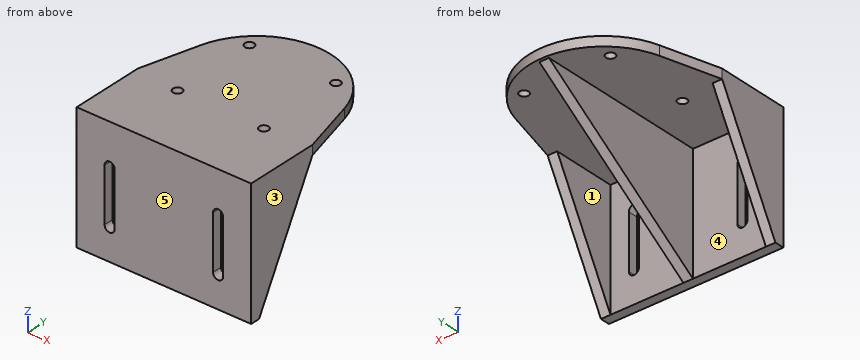
```python
from build123d import *

# Parameters (mm, degrees)
SKETCH_1_R           = 1.447765
EXTRUDE_1_DEPTH      = 3
SKETCH_2_W           = 54.999996422
SKETCH_2_H           = 3
EXTRUDE_2_DEPTH      = 37
CUT_EXTRUDE_1_DEPTH  = 3
EXTRUDE_3_DEPTH      = 3
EXTRUDE_4_DEPTH      = 1.5
EXTRUDE_4_DEPTH_BACK = 1.5


with BuildPart() as part:
    # 草图1 → 凸台-拉伸1 (new body)
    with BuildSketch(Plane.XY):
        with BuildLine():
            Line((-13.887998211, -25.578349272), (-13.887998211, -48.743989272))
            Line((-13.887998211, -48.743989272), (41.111998211, -48.743989272))
            Line((41.111998211, -48.743989272), (41.111998211, -25.578349272))
            Line((41.111998211, -25.578349272), (36.311256918, -7.661738854))
            ThreePointArc((36.311256918, -7.661738854), (13.612, 9.756013586), (-9.087256918, -7.661738854))
            Line((-9.087256918, -7.661738854), (-13.887998211, -25.578349272))
        make_face()
        Circle(SKETCH_1_R, mode=Mode.SUBTRACT)
        with Locations((27.224, 0)):
            Circle(SKETCH_1_R, mode=Mode.SUBTRACT)
        with Locations((0, -27.224)):
            Circle(SKETCH_1_R, mode=Mode.SUBTRACT)
        with Locations((27.224, -27.224)):
            Circle(SKETCH_1_R, mode=Mode.SUBTRACT)
    extrude(amount=-EXTRUDE_1_DEPTH)

    # 草图2 → 凸台-拉伸2 (add)
    with BuildSketch(Plane(origin=(0, 0, -3), x_dir=(-1, 0, 0), z_dir=(0, 0, -1))):
        with Locations((-13.612, -47.243989272)):
            Rectangle(SKETCH_2_W, SKETCH_2_H)
    extrude(amount=EXTRUDE_2_DEPTH)

    # 草图3 → 切除-拉伸1 (cut)
    with BuildSketch(Plane(origin=(0, -45.743989272, 0), x_dir=(1, 0, 0), z_dir=(0, 1, 0))):
        with BuildLine():
            Line((32.311998211, 13), (32.311998211, 30))
            ThreePointArc((32.311998211, 30), (30.711998211, 31.6), (29.111998211, 30))
            Line((29.111998211, 30), (29.111998211, 13))
            ThreePointArc((29.111998211, 13), (30.711998211, 11.4), (32.311998211, 13))
        make_face()
        with BuildLine():
            Line((-1.887998211, 30), (-1.887998211, 13))
            ThreePointArc((-1.887998211, 13), (-3.487998211, 11.4), (-5.087998211, 13))
            Line((-5.087998211, 13), (-5.087998211, 30))
            ThreePointArc((-5.087998211, 30), (-3.487998211, 31.6), (-1.887998211, 30))
        make_face()
    extrude(amount=-CUT_EXTRUDE_1_DEPTH, mode=Mode.SUBTRACT)

    # 草图4 → 凸台-拉伸3 (add)
    with BuildSketch(Plane(origin=(41.111998211, 0, 0), x_dir=(0, 0, -1), z_dir=(1, 0, 0))):
        Polygon((40, -45.743989272), (3, -25.578345661), (3, -45.743989272), align=None)
    extrude_3 = extrude(amount=-EXTRUDE_3_DEPTH)

    # 草图13 → 凸台-拉伸4 (add, two sides: drawn at the far end of the back side and taken through both)
    with BuildSketch(Plane(origin=(13.612, 0, 0), x_dir=(0, 1, 0), z_dir=(-1, 0, 0)).offset(-EXTRUDE_4_DEPTH_BACK)):
        Polygon((-45.743989272, 40), (8.756018173, 3), (-45.743989272, 3), align=None)
    extrude(amount=EXTRUDE_4_DEPTH + EXTRUDE_4_DEPTH_BACK)

    # 镜向1: 凸台-拉伸3 across plane
    add(extrude_3.mirror(Plane.ZY.offset(-13.612)))


solid = part.part
```
Can you work these out from the model? Positions are in its coordinate system, mm. Face numbers are marked on the shaded views. A direction names the side the tool comes from. Coordinates: 2 decimals unless noted, no trailing zeros. Write each loop counter-clockwise with the first axis right and the second up, starting at its lowest first coordinate (ties: lowest second). Pieces come first, ordered by that corner, then holes. Notation, with made-up numbers: (77, 1) - (114, 1) arc R37 ccw to (114, 39) - close; hole circle Ø9 at (22, 80.5). An arc over 180 degrees is marked (long way). Return JSON: item names as keys, results as strings.
Q1. I'm going to push flat-ended pins straight in: pin 1 Ø10 at (x, z) = (25, -29) entering from +Y; pin 2 Ø10 at (y, z) = (-23.5, -4.5) entering from -X; pin 3 Ø2.5 at (x, y) = (0, 0) entering from -Z; pin 4 Ø1.5 at (x, z) = (14, -33) entering from +Y. Where does each tip first touch, or does it pass through?
Computed values:
{"pin 1": "stops at y = -45.74", "pin 2": "stops at x = -13.89", "pin 3": "passes through", "pin 4": "stops at y = -34.33"}
Q2. If we section it at B-B (z = -25): Please give me the cut outline in (x, y).
Computed values:
{"outline": "(-13.89, -48.74) - (-5.09, -48.74) - (-5.09, -45.74) - (-10.89, -45.74) - (-10.89, -37.57) - (-13.89, -37.57) - close; (-1.89, -48.74) - (29.11, -48.74) - (29.11, -45.74) - (15.11, -45.74) - (15.11, -23.65) - (12.11, -23.65) - (12.11, -45.74) - (-1.89, -45.74) - close; (32.31, -48.74) - (41.11, -48.74) - (41.11, -37.57) - (38.11, -37.57) - (38.11, -45.74) - (32.31, -45.74) - close"}
Q3. On a 3-axis mill with a long thin cutter (end or side, diameter ignored), from which of +Z, -Z, +X, -X, +Y, -Y can I reach the whole of each face in a straight line? I mean the marked faces 1 and 2. Say none if no direction works.
Computed values:
{"face 1": "-Z, +Y", "face 2": "+Z, +X, -X, +Y, -Y"}
Q4. If we section it at A-A (x = 0): Please give me the cut outline in (y, z), then the cut area to 3 significant figures.
Computed values:
{"outline": "(-48.74, -40) - (-45.74, -40) - (-45.74, -3) - (-28.67, -3) - (-28.67, 0) - (-48.74, 0) - close; (-25.78, -3) - (-1.45, -3) - (-1.45, 0) - (-25.78, 0) - close; (1.45, -3) - (5.41, -3) - (5.41, 0) - (1.45, 0) - close", "area": "256 mm2"}
Q5. If we section it at D-D (y = 0): Please give me the cut outline in (x, z).
Computed values:
{"outline": "(-5.45, -3) - (-1.45, -3) - (-1.45, 0) - (-5.45, 0) - close; (1.45, -3) - (12.11, -3) - (12.11, -8.94) - (15.11, -8.94) - (15.11, -3) - (25.78, -3) - (25.78, 0) - (1.45, 0) - close; (28.67, -3) - (32.67, -3) - (32.67, 0) - (28.67, 0) - close"}
Q6. Please list where these lines run through material, in increasing order: L1, parallel to X at y = -39.5, z = -22; L2, parallel to Y at x = 17, z = -23; L3, parallel to Z at x = -2, y = -23. Write a range as from..to.
Computed values:
{"L1": "x = -13.89..-10.89, 12.11..15.11, 38.11..41.11", "L2": "y = -48.74..-45.74", "L3": "z = -3..0"}
Q7. If we section it at C-C (y = -23.5): Please give me the cut outline in (x, z).
Computed values:
{"outline": "(-13.33, -3) - (12.11, -3) - (12.11, -24.9) - (15.11, -24.9) - (15.11, -3) - (40.56, -3) - (40.56, 0) - (-13.33, 0) - close"}
Q8. Thinking about a two-plate mould opening in X: for the marked faces 3, 4 and 5, which applies, +X half, -X half, draft (parallel to the pull), parting line (faces both ways), or undercut?
Computed values:
{"face 3": "+X half", "face 4": "undercut", "face 5": "draft"}
